from build123d import *

# Parameters (mm, degrees)
SKETCH1_W          = 304.8
SKETCH1_H          = 142.24
EXTRUDE1_DEPTH     = 2.032
SKETCH3_R          = 1.5875
CUT_EXTRUDE1_DEPTH = 252.699806613
SKETCH4_R          = 7.14375
SKETCH4_R_2        = 1.5875
SKETCH4_R_3        = 3.175
SKETCH4_R_4        = 5.842
EXTRUDE2_DEPTH     = 252.699806613


with BuildPart() as part:
    # Sketch1 → Extrude1 (new body)
    with BuildSketch(Plane.XY):
        with Locations((55.245, 71.12)):
            Rectangle(SKETCH1_W, SKETCH1_H)
    extrude(amount=EXTRUDE1_DEPTH)

    # Sketch3 → Cut-Extrude1 (cut, through all)
    with BuildSketch(Plane.XY.offset(2.032)):
        with Locations((-90.805, 135.89)):
            Circle(SKETCH3_R)
        with Locations((-90.805, 6.35)):
            Circle(SKETCH3_R)
        with Locations((6.35, 135.89)):
            Circle(SKETCH3_R)
        with Locations((6.35, 6.35)):
            Circle(SKETCH3_R)
        with Locations(Location((104.14, 6.35, 0), (0, 0, 180))):
            Circle(SKETCH3_R)
        with Locations(Location((104.14, 135.89, 0), (0, 0, 180))):
            Circle(SKETCH3_R)
        with Locations(Location((201.295, 6.35, 0), (0, 0, 180))):
            Circle(SKETCH3_R)
        with Locations(Location((201.295, 135.89, 0), (0, 0, 180))):
            Circle(SKETCH3_R)
    extrude(amount=-CUT_EXTRUDE1_DEPTH, mode=Mode.SUBTRACT)

    # Sketch4 → Extrude2 (cut, through all)
    with BuildSketch(Plane.XY.offset(2.032)):
        with Locations((-63.8175, 74.6125)):
            Circle(SKETCH4_R)
        with Locations((-39.9415, 74.6125)):
            Circle(SKETCH4_R)
        with Locations((-16.0655, 74.6125)):
            Circle(SKETCH4_R)
        with Locations((-43.18, 137.16)):
            Circle(SKETCH4_R_2)
        with Locations((-9.7155, 47.9425)):
            Circle(SKETCH4_R_3)
        with Locations((-78.105, 19.05)):
            Circle(SKETCH4_R_2)
        with Locations((-29.083, 19.05)):
            Circle(SKETCH4_R_2)
        with Locations((177.165, 104.14)):
            Circle(SKETCH4_R_4)
    extrude(amount=-EXTRUDE2_DEPTH, mode=Mode.SUBTRACT)


solid = part.part
Geometry: final body of the model. Coordinates: model frame, mm. Coordinates: 2 decimals unless noted, no trailing zeros. Order: outer loops, then holes, each group sorted by start corner. A loop starts at its lowest first (then second) coordinate and runs counter-clockwise, first axis right, second up.
1) Section B-B (z = 0.55). Give the number of separate pieces and of enclosed holes in the cut face, then the cut area to 3 significant figures.
Result sheet:
separate pieces: 1
enclosed holes: 16
area: 42,600 mm2
2) Ray query, probe 1 along Y at (x, z) = (6.35, 1); probe 2 along X at (y, z) = (48, 0.65) (3 decimals); probe 3 along X at (y, z) = (135.89, 1.45) (1 decimal). Return the intervals inside material, ascending.
Result sheet:
probe 1: y = 0 to 4.76, 7.94 to 134.3, 137.48 to 142.24
probe 2: x = -97.155 to -12.89, -6.541 to 207.645
probe 3: x = -97.2 to -92.4, -89.2 to -44.1, -42.2 to 4.8, 7.9 to 102.6, 105.7 to 199.7, 202.9 to 207.6
3) Section A-A (y = 78.5). Return loops of the section in (x, z) (3 decimals).
Result sheet:
outline: (-97.155, 0) - (-69.811, 0) - (-69.811, 2.032) - (-97.155, 2.032) - close; (-57.824, 0) - (-45.935, 0) - (-45.935, 2.032) - (-57.824, 2.032) - close; (-33.948, 0) - (-22.059, 0) - (-22.059, 2.032) - (-33.948, 2.032) - close; (-10.072, 0) - (207.645, 0) - (207.645, 2.032) - (-10.072, 2.032) - close
4) Draft query along Y for faces 1 (the cylindrical face through (-8.01, 50.62, 1.03)), 2 (the cylindrical face through (-9.252, 76.758, 1.03)), 3 (the flat face through (53, 72, 0)). Return one class per face: released by +Y, released by -Y, zero draft, split by the parting line, or undercut.
Result sheet:
face 1: undercut
face 2: undercut
face 3: zero draft
5) First-contact query: P1, Ø23, axis at x = -63.82, y = 74.61, coming from the -Z side. Flat tip, straight axial feed; report the tip coordinate or a pass-through.
Result sheet:
P1: stops at z = 0
